The drawing under review shows one solid part. Ordinate dimensions are in mm from its lowest x, y, z. Coordinates: 2 decimals unless noted, no trailing zeros. Write each loop counter-clockwise with the first axis right and the second up, starting at its lowest first coordinate (ties: lowest second). Pieces come first, ordered by that corner, then holes. Notation, with made-up numbers: (6.5, 31) -> (10.5, 31) arc R36 cw to (10.5, 65) -> close; hole circle Ø7 at (-11, -24.75). An arc over 180 degrees is marked (long way). Put each result on its own line as item: value. Start each with the question number.
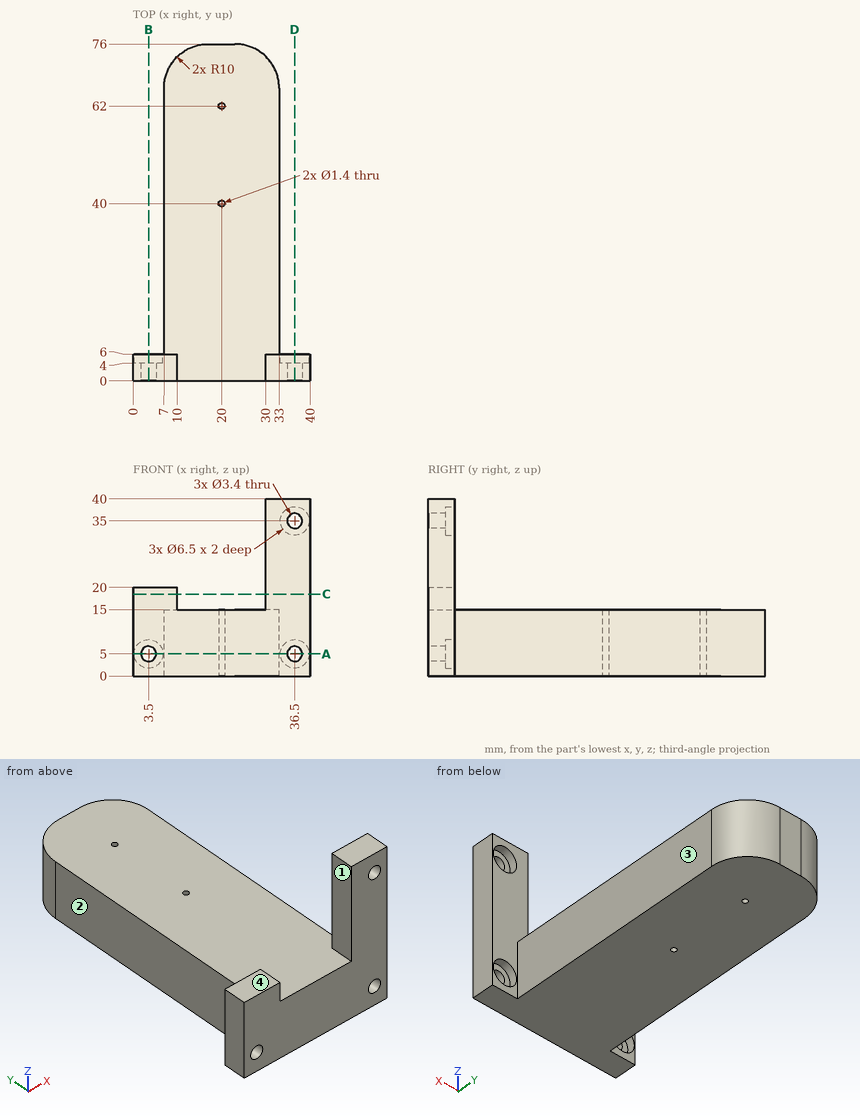
1. The part is to be moulded in two halves that separate along X. For the marked faces 1, 2, 3 and 4, say which applies: released by +X, released by -X, zero draft, split by the parting line, or undercut.
2. Consider section C-C on z = 18.5. State the section outline as (x, y) points, then the cut area to 3 significant figures.
3. Consider section A-A on z = 5. State the section outline as (x, y) points.
4. Wall thickness on line 1 (Y direction, x = 20, z = 5.75); line 2 (X direction, y = 2, z = 5); line 3 (X direction, y = 1.65, z = 35): over which ranges is each line inside the solid? List them lowest first. Write a range as from..to.
5. Consider section D-D on x = 36.5. State the section outline as (y, z) points.
6. Consider section B-B on x = 3.5. State the section outline as (y, z) points.
7. Insertion check: P1, Ø12, axis at x = 31.5, z = 14.5, coming from the +Y side; P2, Ø12, axis at x = 26, y = 15, coming from the +Z side; P3, Ø3, axis at y = 3, z = 23.5, coming from the -X side. Each pin has a flat end and moves straight along its axis. Give the tip position at first contact, or say it passes through.
Output values:
1. face 1: undercut
1. face 2: released by -X
1. face 3: released by +X
1. face 4: zero draft
2. outline: (0, 0) -> (10, 0) -> (10, 6) -> (0, 6) -> close; (30, 0) -> (40, 0) -> (40, 6) -> (30, 6) -> close
2. area: 120 mm^2
3. outline: (0, 0) -> (1.8, 0) -> (1.8, 4) -> (0.25, 4) -> (0.25, 6) -> (0, 6) -> close; (5.2, 0) -> (34.8, 0) -> (34.8, 4) -> (33.25, 4) -> (33.25, 6) -> (33, 6) -> (33, 66) arc R10 ccw to (23, 76) -> (17, 76) arc R10 ccw to (7, 66) -> (7, 6) -> (6.75, 6) -> (6.75, 4) -> (5.2, 4) -> close; (38.2, 0) -> (40, 0) -> (40, 6) -> (39.75, 6) -> (39.75, 4) -> (38.2, 4) -> close; hole circle Ø1.4 at (20, 40); hole circle Ø1.4 at (20, 62)
4. line 1: y = 0..39.3, 40.7..61.3, 62.7..76
4. line 2: x = 0..1.8, 5.2..34.8, 38.2..40
4. line 3: x = 30..34.8, 38.2..40
5. outline: (0, 0) -> (6, 0) -> (6, 1.75) -> (4, 1.75) -> (4, 3.3) -> (0, 3.3) -> close; (0, 6.7) -> (4, 6.7) -> (4, 8.25) -> (6, 8.25) -> (6, 31.75) -> (4, 31.75) -> (4, 33.3) -> (0, 33.3) -> close; (0, 36.7) -> (4, 36.7) -> (4, 38.25) -> (6, 38.25) -> (6, 40) -> (0, 40) -> close
6. outline: (0, 0) -> (6, 0) -> (6, 1.75) -> (4, 1.75) -> (4, 3.3) -> (0, 3.3) -> close; (0, 6.7) -> (4, 6.7) -> (4, 8.25) -> (6, 8.25) -> (6, 20) -> (0, 20) -> close
7. P1: stops at y = 75.68
7. P2: stops at z = 15
7. P3: stops at x = 30
